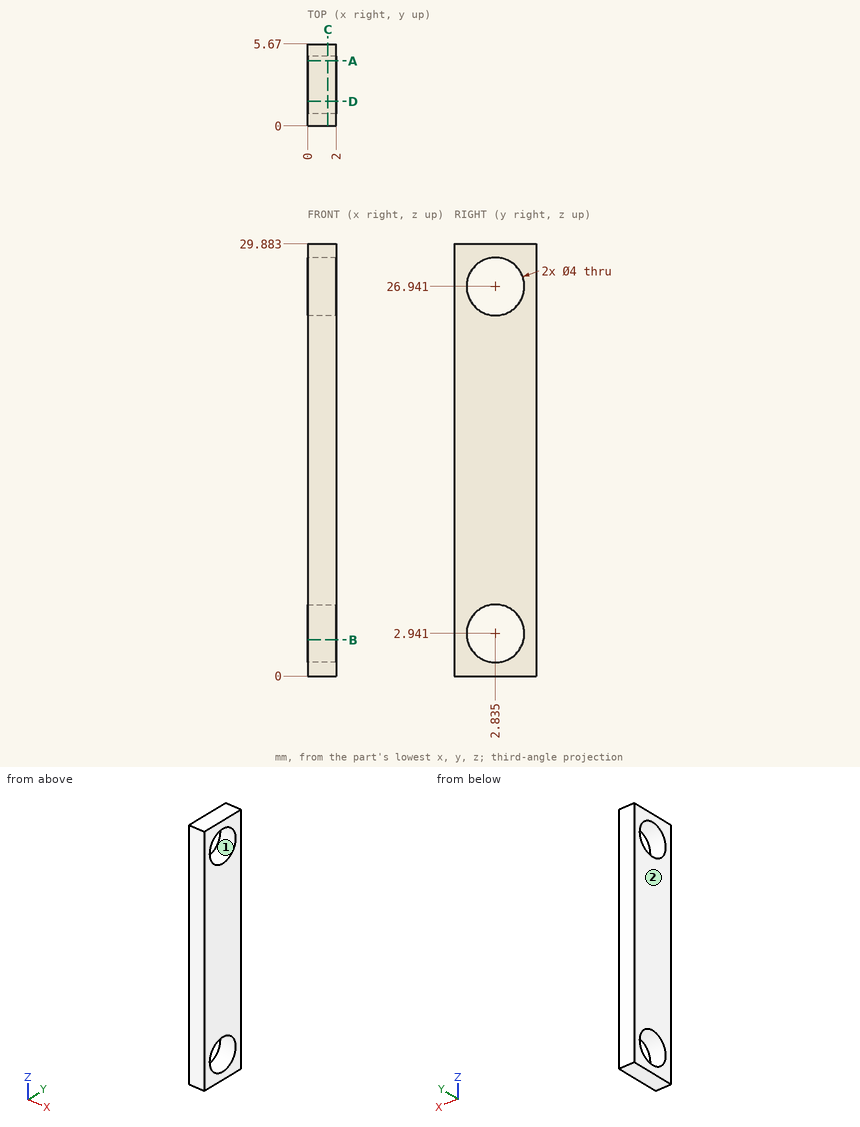
Could you check a few things on this drawing? It's one solid part, dimensions in mm from its lowest x, y, z. Round coordinates to 2 decimals unless told otherwise and drop trailing zeros. Loops run counter-clockwise (first coordinate to the right, second up) from the corner with the lowest first, then second, coordinate; pieces in that order, holes last.
Q1. Thinking about a two-plate mould opening in Y: for the marked faces 1 and 2, which applies, pulls with the +Y half, pulls with the -Y half, needs draft (parallel to the pull), parting line crosses it, or undercut?
Q2. I want a section at B-B (z = 2.5). Write out the boundary of the cut face in (x, y) (1 decimal).
Q3. I want a section at C-C (x = 1.4). Write out the boundary of the cut face in (y, z) (1 decimal).
Q4. Please list where these lines run through material, in increasing order: L1, parallel to Z at x = 1.1, y = 3.65 (1 decimal); L2, parallel to Z at x = 0.95, y = 2.55; L3, parallel to Y at x = 1.05, z = 26.
Q5. I want a section at A-A (y = 4.5). Write out the boundary of the cut face in (x, z).
Q6. I want a section at D-D (y = 1.7). Write out the boundary of the cut face in (x, z) (1 decimal).
Answer below:
1. face 1: undercut
1. face 2: needs draft
2. outline: (0, 0) - (2, 0) - (2, 0.9) - (0, 0.9) - close; (0, 4.8) - (2, 4.8) - (2, 5.7) - (0, 5.7) - close
3. outline: (0, 0) - (5.7, 0) - (5.7, 29.9) - (0, 29.9) - close; hole circle Ø4 at (2.8, 2.9); hole circle Ø4 at (2.8, 26.9)
4. L1: z = 0 to 1.1, 4.8 to 25.1, 28.8 to 29.9
4. L2: z = 0 to 0.96, 4.92 to 24.96, 28.92 to 29.88
4. L3: y = 0 to 1.07, 4.6 to 5.67
5. outline: (0, 0) - (2, 0) - (2, 1.83) - (0, 1.83) - close; (0, 4.05) - (2, 4.05) - (2, 25.83) - (0, 25.83) - close; (0, 28.05) - (2, 28.05) - (2, 29.88) - (0, 29.88) - close
6. outline: (0, 0) - (2, 0) - (2, 1.3) - (0, 1.3) - close; (0, 4.6) - (2, 4.6) - (2, 25.3) - (0, 25.3) - close; (0, 28.6) - (2, 28.6) - (2, 29.9) - (0, 29.9) - close
